For this review, take the finished solid that the model builds, in its own axes (mm). A direction names the side the tool comes from. Coordinates: 2 decimals unless noted, no trailing zeros. Order: outer loops, then holes, each group sorted by start corner. A loop starts at its lowest first (then second) coordinate and runs counter-clockwise, first axis right, second up. Notation, with made-up numbers: (15, 43.5) -> (45, 43.5) arc R10 cw to (45, 60.5) -> close; hole circle Ø7 at (74, 41.5). An arc over 180 degrees is marked (long way). Return JSON: item names as keys, results as strings. Group by question number.
Item 1: Take a section at C-C (z = -32.5). Write out the cut boundary in (x, y), then the cut area to 3 significant figures.
Item 2: Take a section at D-D (y = -1.5). Write out the cut boundary in (x, z).
Item 3: Draft analysis for pull direction X (two halves, no side actions). For faces 5 (the flat face through (102.5, -2, -316)), 6 (the flat face through (-72.5, 41, -163)), 7 (the flat face through (-85, -7.5, -177)), state which applies: +X half, -X half, draft (parallel to the pull), parting line (faces both ways), or undercut.
Item 4: Insertion check: pin 1 (2 mm diameter, centred on y = 53.5, z = -207, fed in from -X); pin 2 (8 mm diameter, centred on y = -20, z = -92.5, fed in from -X); pin 3 (6 mm diameter, centred on x = -45, z = -194.5, fed in from +Y). Each pin has a flat end and moves straight along its axis. Give the tip position at first contact, or say it passes through.
Item 5: Machinability: for faces 1 (the flat face through (72.5, 39, -163)), 2 (the flat face through (162.5, -17, -314)), 3 (the flat face through (172.5, -23, -177)), 4 (the flat face through (51, -7.5, -177)), which of the approach directions +Z, -Z, +X, -X, +Y, -Y give a long, thin tool a straight path to every point of the face, cutting with its end or side? Answer none if there is none.
Item 6: Take a section at A-A (y = -19.5). Write out the cut boundary in (x, z).
Item 7: Take a section at B-B (z = -315). Write out the cut boundary in (x, y).
Item 8: For line 1 along X through (y, z) = (-14, -214); line 2 along Y through (x, z) = (128.5, -124); line 3 along X through (y, z) = (46, -257.5), list the stretches that pass through material, from the lowest coordinate up.
```python
from build123d import *

# Parameters (mm, degrees)
BOSS_EXTRUDE1_DEPTH = 360
CUT_EXTRUDE1_DEPTH  = 360
SKETCH4_W           = 30
SKETCH4_H           = 75
CUT_EXTRUDE2_DEPTH  = 276


with BuildPart() as part:
    # Sketch1 → Boss-Extrude1 (new body)
    with BuildSketch(Plane.XY):
        with BuildLine():
            Line((-72.5, 2.5), (-102.5, 2.5))
            Line((-102.5, 2.5), (-102.5, -7.5))
            Line((-102.5, -7.5), (-67.5, -7.5))
            Line((-67.5, -7.5), (-67.5, -37.5))
            Line((-67.5, -37.5), (-57.5, -37.5))
            Line((-57.5, -37.5), (-57.5, -7.5))
            Line((-57.5, -7.5), (57.5, -7.5))
            Line((57.5, -7.5), (67.5, -7.5))
            Line((67.5, -7.5), (162.5, -7.5))
            Line((162.5, -7.5), (162.5, -37.5))
            Line((162.5, -37.5), (172.5, -37.5))
            Line((172.5, -37.5), (172.5, -7.5))
            Line((172.5, -7.5), (202.5, -7.5))
            Line((202.5, -7.5), (202.5, 2.5))
            Line((202.5, 2.5), (72.5, 2.5))
            Line((72.5, 2.5), (72.5, 77.5))
            ThreePointArc((72.5, 77.5), (0, 5), (-72.5, 77.5))
            Line((-72.5, 77.5), (-72.5, 2.5))
        make_face()
    extrude(amount=-BOSS_EXTRUDE1_DEPTH)

    # Sketch3 → Cut-Extrude1 (cut)
    with BuildSketch(Plane(origin=(0, 2.5, 0), x_dir=(1, 0, 0), z_dir=(0, 1, 0))):
        with BuildLine():
            Line((102.5, 360), (102.5, 270))
            ThreePointArc((102.5, 270), (132.5, 239.895652489), (162.5, 270))
            Line((162.5, 270), (162.5, 360))
            Line((162.5, 360), (102.5, 360))
        make_face()
    extrude(amount=-CUT_EXTRUDE1_DEPTH, mode=Mode.SUBTRACT)

    # Sketch4 → Cut-Extrude2 (cut, through all)
    with BuildSketch(Plane.ZY.offset(72.5)):
        with Locations((-345, 40)):
            Rectangle(SKETCH4_W, SKETCH4_H)
    extrude(amount=-CUT_EXTRUDE2_DEPTH, mode=Mode.SUBTRACT)


solid = part.part
```
Findings below:
{
 "1": {"outline": "(-102.5, -7.5) -> (-67.5, -7.5) -> (-67.5, -37.5) -> (-57.5, -37.5) -> (-57.5, -7.5) -> (162.5, -7.5) -> (162.5, -37.5) -> (172.5, -37.5) -> (172.5, -7.5) -> (202.5, -7.5) -> (202.5, 2.5) -> (72.5, 2.5) -> (72.5, 77.5) arc R72.5 cw to (-72.5, 77.5) -> (-72.5, 2.5) -> (-102.5, 2.5) -> close", "area": "6,270 mm2"},
 "2": {"outline": "(-102.5, -360) -> (102.5, -360) -> (102.5, -270) arc R30 cw (long way) to (162.5, -270) -> (162.5, -360) -> (202.5, -360) -> (202.5, 0) -> (-102.5, 0) -> close"},
 "3": {"face 5": "undercut", "face 6": "-X half", "face 7": "draft"},
 "4": {"pin 1": "stops at x = -72.5", "pin 2": "stops at x = -67.5", "pin 3": "stops at y = 23.17"},
 "5": {"face 1": "+Z, -Z, +X, +Y", "face 2": "-Z, +Y, -Y", "face 3": "+Z, -Z, +X, -Y", "face 4": "+Z, -Z, -Y"},
 "6": {"outline": "(-67.5, -360) -> (-57.5, -360) -> (-57.5, 0) -> (-67.5, 0) -> close; (162.5, -360) -> (172.5, -360) -> (172.5, 0) -> (162.5, 0) -> (162.5, -269.79) arc R30 cw to (162.5, -270) -> close"},
 "7": {"outline": "(-102.5, -7.5) -> (-67.5, -7.5) -> (-67.5, -37.5) -> (-57.5, -37.5) -> (-57.5, -7.5) -> (102.5, -7.5) -> (102.5, 2.5) -> (72.5, 2.5) -> (72.5, 77.5) arc R72.5 cw to (-72.5, 77.5) -> (-72.5, 2.5) -> (-102.5, 2.5) -> close; (162.5, -37.5) -> (172.5, -37.5) -> (172.5, -7.5) -> (202.5, -7.5) -> (202.5, 2.5) -> (162.5, 2.5) -> close"},
 "8": {"line 1": "x = -67.5 to -57.5, 162.5 to 172.5", "line 2": "y = -7.5 to 2.5", "line 3": "x = -72.5 to -65.3, 65.3 to 72.5"}
}
